The listing builds one solid part. Answer for the finished solid, in the listing's coordinates (mm). Coordinates: 2 decimals unless noted, no trailing zeros. Order: outer loops, then holes, each group sorted by start corner. A loop starts at its lowest first (then second) coordinate and runs counter-clockwise, first axis right, second up. Notation, with made-up numbers: (-0.75, 43) - (35.25, 43) arc R7 cw to (35.25, 48) - close; hole circle Ø1 at (21, 67). An arc over 180 degrees is marked (long way). One line per item, written item: value. Start each with the question number.
```python
from build123d import *

# Parameters (mm, degrees)
SKETCH_1_R               = 156
EXTRUDE_1_DEPTH          = 8
SKETCH_5_R               = 6
CUT_EXTRUDE_4_DEPTH      = 10
PATTERN_CIRCULAR_3_COUNT = 4
SKETCH_6_W               = 86
SKETCH_6_H               = 86
CUT_EXTRUDE_5_DEPTH      = 10
SKETCH_7_R               = 7
CUT_EXTRUDE_6_DEPTH      = 10


with BuildPart() as part:
    # 草图1 → 凸台-拉伸1 (new body)
    with BuildSketch(Plane(origin=(0, 0, 0), x_dir=(0, 0, -1), z_dir=(1, 0, 0))):
        Circle(SKETCH_1_R)
    extrude(amount=EXTRUDE_1_DEPTH)

    # 草图5 → 切除-拉伸4 (cut)
    with BuildSketch(Plane(origin=(8, 0, 0), x_dir=(0, 0, -1), z_dir=(1, 0, 0))):
        with Locations((0, 130)):
            Circle(SKETCH_5_R)
    cut_extrude_4 = extrude(amount=-CUT_EXTRUDE_4_DEPTH, mode=Mode.SUBTRACT)

    # 阵列(圆周)3: 切除-拉伸4 ×4 about axis
    pattern_circular_3_axis = Axis((0, 0, 0), (1, 0, 0))
    for i in range(1, PATTERN_CIRCULAR_3_COUNT):
        add(cut_extrude_4.rotate(pattern_circular_3_axis, i * 360 / PATTERN_CIRCULAR_3_COUNT), mode=Mode.SUBTRACT)

    # 草图6 → 切除-拉伸5 (cut)
    with BuildSketch(Plane(origin=(8, 0, 0), x_dir=(0, 0, -1), z_dir=(1, 0, 0))):
        Rectangle(SKETCH_6_W, SKETCH_6_H)
    extrude(amount=-CUT_EXTRUDE_5_DEPTH, mode=Mode.SUBTRACT)

    # 草图7 → 切除-拉伸6 (cut)
    with BuildSketch(Plane(origin=(8, 0, 0), x_dir=(0, 0, -1), z_dir=(1, 0, 0))):
        with Locations((0, 80)):
            Circle(SKETCH_7_R)
        with Locations((0, -80)):
            Circle(SKETCH_7_R)
    extrude(amount=-CUT_EXTRUDE_6_DEPTH, mode=Mode.SUBTRACT)


solid = part.part
```
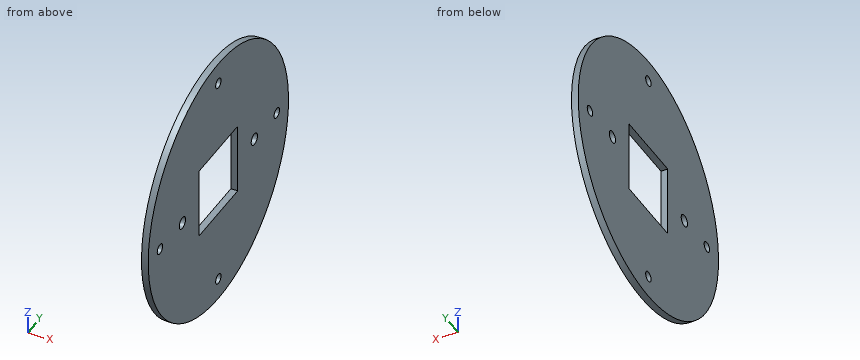
(1) Flat-ended cylindrical pins translate along their axes: pin 1 Ø8.5 at (y, z) = (-80, 0) entering from -X; pin 2 Ø2.5 at (x, z) = (5, 10) entering from +Y; pin 3 Ø2.5 at (x, z) = (2.5, 15) entering from -Y; pin 4 Ø2.5 at (x, y) = (2, -8) entering from -Z. Find the tip coordinate at first contact, or state that the pin passes through.
(2) Consider probe 1 along Y at (x, z) = (3.5, 0); probe 2 along Y at (x, z) = (2, -2); probe 3 along Z at (x, y) = (5.5, -130). Determine where each line is inside the solid, lowest interval first.
(3) The part is cut by section B-B on y = 16. Determine the outline of the cut face in (x, z), plus the area to 3 significant figures.
(4) The part is cut by section D-D on z = 130. Determine the outline of the cut face in (x, y), plus the area to 3 significant figures.
(5) The part is cut by section C-C on x = 4. Determine the outline of the cut face in (y, z), plus the area to 3 significant figures.
(6) The part is cut by section A-A on z = 0. Determine the outline of the cut face in (x, y).
Completed:
1. pin 1: passes through
1. pin 2: stops at y = 155.75
1. pin 3: stops at y = -155.39
1. pin 4: stops at z = -155.85
2. probe 1: y = -156 to -136, -124 to -87, -73 to -43, 43 to 73, 87 to 124, 136 to 156
2. probe 2: y = -155.99 to -135.66, -124.34 to -86.71, -73.29 to -43, 43 to 73.29, 86.71 to 124.34, 135.66 to 155.99
2. probe 3: z = -86.23 to -6, 6 to 86.23
3. outline: (0, -155.18) - (8, -155.18) - (8, -43) - (0, -43) - close; (0, 43) - (8, 43) - (8, 155.18) - (0, 155.18) - close
3. area: 1,790 mm2
4. outline: (0, -86.23) - (8, -86.23) - (8, -6) - (0, -6) - close; (0, 6) - (8, 6) - (8, 86.23) - (0, 86.23) - close
4. area: 1,280 mm2
5. outline: circle Ø312 at (0, 0); hole circle Ø12 at (-130, 0); hole circle Ø14 at (-80, 0); hole (-43, -43) - (43, -43) - (43, 43) - (-43, 43) - close; hole circle Ø12 at (0, -130); hole circle Ø12 at (0, 130); hole circle Ø14 at (80, 0); hole circle Ø12 at (130, 0)
5. area: 68,300 mm2
6. outline: (0, -156) - (8, -156) - (8, -136) - (0, -136) - close; (0, -124) - (8, -124) - (8, -87) - (0, -87) - close; (0, -73) - (8, -73) - (8, -43) - (0, -43) - close; (0, 43) - (8, 43) - (8, 73) - (0, 73) - close; (0, 87) - (8, 87) - (8, 124) - (0, 124) - close; (0, 136) - (8, 136) - (8, 156) - (0, 156) - close
